Read the model definition and answer for the solid it produces. Units are mm, in the model's axes. A direction names the side the tool comes from. Coordinates: 2 decimals unless noted, no trailing zeros. Loops run counter-clockwise (first coordinate to the right, second up) from the corner with the lowest first, then second, coordinate; pieces in that order, holes last.
from build123d import *

# Parameters (mm, degrees)
F0_R     = 5
F1_DEPTH = 4
F2_DEPTH = 25
F3_R     = 6


with BuildPart() as f1:
    # F0 (on Front) → F1 (new body)
    with BuildSketch(Plane.XZ):
        with BuildLine():
            Line((-20.45353, 41.072611), (-65.051813, 91.24568))
            ThreePointArc((-65.051813, 91.24568), (-89.965457, 101.21114), (-82.989636, 75.30095))
            Line((-82.989636, 75.30095), (-35.262953, 21.608432))
            ThreePointArc((-35.262953, 21.608432), (-34.326391, 20.063516), (-34, 18.286613))
            Line((-34, 18.286613), (-34, -18.286613))
            ThreePointArc((-34, -18.286613), (-34.326391, -20.063516), (-35.262953, -21.608432))
            Line((-35.262953, -21.608432), (-82.989636, -75.30095))
            ThreePointArc((-82.989636, -75.30095), (-89.965457, -101.21114), (-65.051813, -91.24568))
            Line((-65.051813, -91.24568), (-20.45353, -41.072611))
            ThreePointArc((-20.45353, -41.072611), (-18.764763, -39.83323), (-16.716483, -39.39443))
            Line((-16.716483, -39.39443), (16.716483, -39.39443))
            ThreePointArc((16.716483, -39.39443), (18.764763, -39.83323), (20.45353, -41.072611))
            Line((20.45353, -41.072611), (65.051813, -91.24568))
            ThreePointArc((65.051813, -91.24568), (89.965457, -101.21114), (82.989636, -75.30095))
            Line((82.989636, -75.30095), (35.262953, -21.608432))
            ThreePointArc((35.262953, -21.608432), (34.326391, -20.063516), (34, -18.286613))
            Line((34, -18.286613), (34, 18.286613))
            ThreePointArc((34, 18.286613), (34.326391, 20.063516), (35.262953, 21.608432))
            Line((35.262953, 21.608432), (82.989636, 75.30095))
            ThreePointArc((82.989636, 75.30095), (89.965457, 101.21114), (65.051813, 91.24568))
            Line((65.051813, 91.24568), (20.45353, 41.072611))
            ThreePointArc((20.45353, 41.072611), (18.764763, 39.83323), (16.716483, 39.39443))
            Line((16.716483, 39.39443), (-16.716483, 39.39443))
            ThreePointArc((-16.716483, 39.39443), (-18.764763, 39.83323), (-20.45353, 41.072611))
        make_face()
        with Locations((-80, -90)):
            Circle(F0_R, mode=Mode.SUBTRACT)
        with Locations((80, -90)):
            Circle(F0_R, mode=Mode.SUBTRACT)
        with Locations((-80, 90)):
            Circle(F0_R, mode=Mode.SUBTRACT)
        with Locations((80, 90)):
            Circle(F0_R, mode=Mode.SUBTRACT)
    extrude(amount=F1_DEPTH)

    # F4 (on face) → F2 (cut)
    with BuildSketch(Plane.XZ.offset(4)):
        with BuildLine():
            ThreePointArc((19.25, 17.5), (17.5, 19.25), (15.75, 17.5))
            Line((15.75, 17.5), (17.5, 17.5))
            Line((17.5, 17.5), (17.5, 15.75))
            ThreePointArc((17.5, 15.75), (18.737437, 16.262563), (19.25, 17.5))
        make_face()
        with BuildLine():
            Line((-17.5, 17.5), (-15.75, 17.5))
            ThreePointArc((-15.75, 17.5), (-18.737437, 18.737437), (-17.5, 15.75))
            Line((-17.5, 15.75), (-17.5, 17.5))
        make_face()
        with BuildLine():
            ThreePointArc((-17.5, 15.75), (-16.262563, 16.262563), (-15.75, 17.5))
            Line((-15.75, 17.5), (-17.5, 17.5))
            Line((-17.5, 17.5), (-17.5, 15.75))
        make_face()
        with BuildLine():
            Line((17.5, 17.5), (15.75, 17.5))
            ThreePointArc((15.75, 17.5), (16.262563, 16.262563), (17.5, 15.75))
            Line((17.5, 15.75), (17.5, 17.5))
        make_face()
        with BuildLine():
            ThreePointArc((-15.75, -17.5), (-16.262563, -16.262563), (-17.5, -15.75))
            Line((-17.5, -15.75), (-17.5, -17.5))
            Line((-17.5, -17.5), (-15.75, -17.5))
        make_face()
        with BuildLine():
            Line((-17.5, -17.5), (-17.5, -15.75))
            ThreePointArc((-17.5, -15.75), (-18.737437, -18.737437), (-15.75, -17.5))
            Line((-15.75, -17.5), (-17.5, -17.5))
        make_face()
        with BuildLine():
            Line((17.5, -17.5), (17.5, -15.75))
            ThreePointArc((17.5, -15.75), (16.262563, -16.262563), (15.75, -17.5))
            Line((15.75, -17.5), (17.5, -17.5))
        make_face()
        with BuildLine():
            ThreePointArc((19.25, -17.5), (18.737437, -16.262563), (17.5, -15.75))
            Line((17.5, -15.75), (17.5, -17.5))
            Line((17.5, -17.5), (15.75, -17.5))
            ThreePointArc((15.75, -17.5), (17.5, -19.25), (19.25, -17.5))
        make_face()
    extrude(amount=-F2_DEPTH, mode=Mode.SUBTRACT)

    # F3
    f3_edges = [f1.edges().sort_by_distance(p)[0] for p in [
        (82.989636, -2, -75.30095),
        (65.051813, -2, -91.24568),
        (-82.989636, -2, -75.30095),
        (-65.051813, -2, -91.24568),
        (65.051813, -2, 91.24568),
        (82.989636, -2, 75.30095),
        (-82.989636, -2, 75.30095),
        (-65.051813, -2, 91.24568),
    ]]
    fillet(f3_edges, radius=F3_R)


solid = f1.part
Q1. Which of the six approach directions +Z, -Z, +X, -X, +Y, -Y give full straight-line access (tool end or side, diameter ignored) to faces 1 (the face through (-41.845, -1.972, 65.139)), 2 (the face through (-58.2, -1.97, -47.41)), 3 (the face through (41.845, -1.972, -65.139)), 4 (the face through (58.848, -1.972, -48.142))?
Findings below:
face 1: +Z, +Y, -Y
face 2: -X, +Y, -Y
face 3: -Z, +Y, -Y
face 4: +X, +Y, -Y
Q2. A cutting plane is placed at D-D (z = 4). Give the vertices of the cut face in (x, y), then the cut area to 3 significant figures.
Findings below:
outline: (-34, -4) - (34, -4) - (34, 0) - (-34, 0) - close
area: 272 mm2
Q3. A cutting plane is placed at B-B (x = -51). Give the vertices of the cut face in (y, z), then the cut area to 3 significant figures.
Findings below:
outline: (-4, -75.44) - (0, -75.44) - (0, -39.31) - (-4, -39.31) - close; (-4, 39.31) - (0, 39.31) - (0, 75.44) - (-4, 75.44) - close
area: 289 mm2
Q4. Straight lines are drawn through the part: probe 1 along X at (y, z) = (-0.95, 17.5); probe 2 along Z at (x, y) = (-80, -2.65); probe 3 along Z at (x, y) = (-79, -1.75). For each, find the intervals that lie inside material, in ascending order.
Findings below:
probe 1: x = -34 to -19.25, -15.75 to 15.75, 19.25 to 34
probe 2: z = -105 to -95, -85 to -71.94, 71.94 to 85, 95 to 105
probe 3: z = -104.97 to -94.9, -85.1 to -70.81, 70.81 to 85.1, 94.9 to 104.97
Q5. A cutting plane is placed at A-A (z = 59). Give the vertices of the cut face in (x, y), then the cut area to 3 significant figures.
Findings below:
outline: (-68.5, -4) - (-36.39, -4) - (-36.39, 0) - (-68.5, 0) - close; (36.39, -4) - (68.5, -4) - (68.5, 0) - (36.39, 0) - close
area: 257 mm2
Q6. Determine the mould class of faces 5 (the face through (0, -4, 0)), 6 (the face through (58.2, -1.97, 47.41)), 7 (the face through (42.45, -1.97, 65.82)) for opening direction X: +X half, -X half, draft (parallel to the pull), parting line (faces both ways), or undercut.
Findings below:
face 5: draft
face 6: +X half
face 7: undercut
Q7. A cutting plane is placed at C-C (y = -1.05). Count the separate pieces of the cut face and the enclosed holes in it, then the cut area to 3 significant figures.
Findings below:
separate pieces: 1
enclosed holes: 8
area: 13,700 mm2
Q8. Flat-ended cylindrical pins translate along their axes: pin 1 Ø2 at (y, z) = (-2, 6) entering from -X; pin 2 Ø6 at (x, z) = (80, 90) entering from +Y; pin 3 Ø2 at (y, z) = (-0.5, -60) entering from +X; pin 4 Ø1.2 at (y, z) = (-2, -1.5) entering from +X. Find the tip coordinate at first contact, or state that the pin passes through.
Findings below:
pin 1: stops at x = -34
pin 2: passes through
pin 3: stops at x = 70.28
pin 4: stops at x = 34
